```python
from build123d import *

# Parameters (mm, degrees)
BOSS_EXTRUDE1_DEPTH = 10
SKETCH2_R           = 10
BOSS_EXTRUDE2_DEPTH = 10


with BuildPart() as part:
    # Sketch1 → Boss-Extrude1 (new body)
    with BuildSketch(Plane(origin=(0, 0, 0), x_dir=(0, 0, -1), z_dir=(1, 0, 0))):
        with BuildLine():
            Line((-19.310323675, 18.90886515), (560.689676325, 18.90886515))
            ThreePointArc((560.689676325, 18.90886515), (567.760744137, 15.979932962), (570.689676325, 8.90886515))
            Line((570.689676325, 8.90886515), (570.689676325, -1.09113485))
            ThreePointArc((570.689676325, -1.09113485), (567.760744137, -8.162202662), (560.689676325, -11.09113485))
            Line((560.689676325, -11.09113485), (-19.310323675, -11.09113485))
            ThreePointArc((-19.310323675, -11.09113485), (-26.381391487, -8.162202662), (-29.310323675, -1.09113485))
            Line((-29.310323675, -1.09113485), (-29.310323675, 8.90886515))
            ThreePointArc((-29.310323675, 8.90886515), (-26.381391487, 15.979932962), (-19.310323675, 18.90886515))
        make_face()
    extrude(amount=BOSS_EXTRUDE1_DEPTH)

    # Sketch2 → Boss-Extrude2 (add)
    with BuildSketch(Plane(origin=(10, 0, 0), x_dir=(0, 0, -1), z_dir=(1, 0, 0))):
        with Locations((-11.135288293, 3.90886515)):
            Circle(SKETCH2_R)
    extrude(amount=BOSS_EXTRUDE2_DEPTH)


solid = part.part
```
Here's how the part is built. I have some questions about the finished solid (model axes, mm). A direction names the side the tool comes from. Give positions to 0.01 mm unless a question says otherwise; leave off trailing zeros. Loops run counter-clockwise (first coordinate to the right, second up) from the corner with the lowest first, then second, coordinate; pieces in that order, holes last. Notation, with made-up numbers: M 5,20.5 L 51,20.5 A22 cw 51,32.5 Z; hole C -7,69 d4. An arc over 180 degrees is marked long. Return JSON: item names as keys, results as strings.
Item 1: Imagine slicing it at B-B on x = 14.75. List the corners of the cut face in (y, z) for me.
A:
{"outline": "C 3.91,11.14 d20"}
Item 2: On a 3-axis mill with a long thin cutter (end or side, diameter ignored), from which of +Z, -Z, +X, -X, +Y, -Y can I reach the whole of each face in a straight line? I mean faces 1 (the cylindrical face through (4.93, 16.06, -567.68)), 2 (the cylindrical face through (14.93, 12.34, 5.76)). Say none if no direction works.
A:
{"face 1": "-Z, +X, -X, +Y", "face 2": "+X"}
Item 3: I'm going to push flat-ended pins straight in: pin 1 Ø1.5 at (x, y) = (17.5, -4) entering from -Z; pin 2 Ø3 at (y, z) = (3.5, -37) entering from +X; pin 3 Ø2 at (x, y) = (3.5, -7.5) entering from -Z. Where does each tip first touch, or does it pass through?
A:
{"pin 1": "stops at z = 4.15", "pin 2": "stops at x = 10", "pin 3": "stops at z = -569.1"}
Item 4: Please list where these lines run through material, in increasing order: line 1 (X direction, y = 3, z = -18); line 2 (Z direction, x = 1.75, y = -7.5); line 3 (Z direction, x = 2, y = -9.5).
A:
{"line 1": "x = 0 to 10", "line 2": "z = -568.37 to 26.99", "line 3": "z = -566.1 to 24.72"}
Item 5: Imagine slicing it at A-A on z = -390. List the corners of the cut face in (x, y) for me, then the cut area to 3 significant figures.
A:
{"outline": "M 0,-11.09 L 10,-11.09 L 10,18.91 L 0,18.91 Z", "area": "300 mm^2"}
